Could you check a few things on this model? Use its own coordinates, in mm. A direction names the side the tool comes from. Round coordinates to 2 decimals unless told otherwise and drop trailing zeros. Loops run counter-clockwise (first coordinate to the right, second up) from the corner with the lowest first, then second, coordinate; pieces in that order, holes last. Notation, with made-up numbers: (40, -10) -> (83, -10) arc R5 ccw to (83, -6) -> close; hole circle Ø1 at (25, 40.25). An arc over 180 degrees is marked (long way). Write each question's results on one line, items separated by ' | '.
from build123d import *

# Parameters (mm, degrees)
F0_R      = 29.21
F10_DEPTH = 19.05
F1_R      = 3.175
F2_DEPTH  = 3.175
F3_R      = 1.5875
F4_DEPTH  = 28.575
F5_R      = 3.175
F11_DEPTH = 9.526
F6_R      = 1.5875
F7_DEPTH  = 25.4
F8_R      = 1.5875
F9_DEPTH  = 25.4


with BuildPart() as f10:
    # F0 (on Top) → F10 (new body)
    with BuildSketch(Plane.XY):
        with BuildLine():
            Line((38.1, 63.5), (-139.7, 63.5))
            ThreePointArc((-139.7, 63.5), (-157.6605122421, 56.0605122421), (-165.1, 38.1))
            Line((-165.1, 38.1), (-165.1, -38.1))
            ThreePointArc((-165.1, -38.1), (-157.6605122421, -56.0605122421), (-139.7, -63.5))
            Line((-139.7, -63.5), (38.1, -63.5))
            ThreePointArc((38.1, -63.5), (56.0605122421, -56.0605122421), (63.5, -38.1))
            Line((63.5, -38.1), (63.5, 6.1400658214))
            ThreePointArc((63.5, 6.1400658214), (63.1105704313, 8.3296091832), (61.9900472022, 10.2505941427))
            Line((61.9900472022, 10.2505941427), (50.937113555, 23.2651548983))
            ThreePointArc((50.937113555, 23.2651548983), (50.192630832, 25.5783429328), (51.3018729955, 27.7404426601))
            Line((51.3018729955, 27.7404426601), (61.058563678, 36.026550563))
            ThreePointArc((61.058563678, 36.026550563), (62.8898833704, 38.6267446044), (63.2307138089, 41.7887970203))
            ThreePointArc((63.2307138089, 41.7887970203), (62.4610549959, 45.2902016304), (61.206100491, 48.648370495))
            Line((61.206100491, 48.648370495), (35.46918169, 26.7906634902))
            ThreePointArc((35.46918169, 26.7906634902), (-34.6889292719, -27.7935367661), (33.8803304154, 28.7736982493))
            Line((33.8803304154, 28.7736982493), (60.0039803909, 50.9598461512))
            ThreePointArc((60.0039803909, 50.9598461512), (50.719823845, 60.1431405685), (38.1, 63.5))
        make_face()
        with Locations((-107.95, 0)):
            Circle(F0_R, mode=Mode.SUBTRACT)
    extrude(amount=F10_DEPTH)

    # F1 (on face) → F2 (cut)
    with BuildSketch(Plane.XY):
        with Locations((-152.4, -50.8)):
            Circle(F1_R)
        with Locations((50.8, -50.8)):
            Circle(F1_R)
        with Locations((50.8, 50.8)):
            Circle(F1_R)
        with Locations((-152.4, 50.8)):
            Circle(F1_R)
    extrude(amount=F2_DEPTH, mode=Mode.SUBTRACT)

    # F3 (on face) → F4 (cut)
    with BuildSketch(Plane(origin=(7.8100038105, -9.1960896842, 0), x_dir=(0.7622121578, 0.6473272947, 0), z_dir=(0.6473272947, -0.7622121578, 0))):
        with Locations((63.4603030527, 9.525)):
            Circle(F3_R)
    extrude(amount=-F4_DEPTH, mode=Mode.SUBTRACT)

    # F5 (on face) → F11 (cut, through all)
    with BuildSketch(Plane(origin=(7.8100038105, -9.1960896842, 0), x_dir=(0.7622121578, 0.6473272947, 0), z_dir=(0.6473272947, -0.7622121578, 0))):
        with Locations((63.4603030527, 9.525)):
            Circle(F5_R)
    extrude(amount=-F11_DEPTH, mode=Mode.SUBTRACT)

    # F6 (on face) → F7 (cut)
    with BuildSketch(Plane.XZ.offset(63.5)):
        with Locations((-108.2258597016, 9.525)):
            Circle(F6_R)
    extrude(amount=-F7_DEPTH, mode=Mode.SUBTRACT)

    # F8 (on face) → F9 (cut)
    with BuildSketch(Plane(origin=(-165.1, 0, 0), x_dir=(0, -1, 0), z_dir=(-1, 0, 0))):
        with Locations((0, 9.525)):
            Circle(F8_R)
    extrude(amount=-F9_DEPTH, mode=Mode.SUBTRACT)


solid = f10.part
1) I need wall thicknesses on line 1 (Y direction, x = -152.4, z = 2.3) (3 decimals); line 2 (X direction, y = 18.5, z = 1.25); line 3 (Z direction, x = -154.5, y = 0). Which ranges of each line are inside material? Lowest first, please.
Model answer:
line 1: y = -60.097 to -53.975, -47.625 to 47.625, 53.975 to 60.097 | line 2: x = -165.1 to -130.55, -85.35 to -40.42, 40.42 to 54.98 | line 3: z = 0 to 7.94, 11.11 to 19.05
2) I'm going to push flat-ended pins straight in: pin 1 (10 mm diameter, centred on x = -152.4, y = -50.8, fed in from -Z); pin 2 (6 mm diameter, centred on x = -29.5, y = -26.5, fed in from -Z); pin 3 (1.6 mm diameter, centred on y = -0.5, z = 9.5, fed in from -X); pin 4 (3 mm diameter, centred on x = -151.5, y = -51.5, fed in from -Z) (3 decimals). Where does each tip first touch, or does it pass through?
Model answer:
pin 1: stops at z = 0 | pin 2: passes through | pin 3: stops at x = -139.7 | pin 4: stops at z = 3.175
3) I want a section at D-D, the plane y = -34.5. Write out the boundary of the cut face in (x, z).
Model answer:
outline: (-165.1, 0) -> (-28.03, 0) -> (-28.03, 19.05) -> (-165.1, 19.05) -> close; (28.03, 0) -> (63.5, 0) -> (63.5, 19.05) -> (28.03, 19.05) -> close
4) If we mould it in two halves opening along X, with no side actions, what happens to faces 1 (the flat face through (-52, 1, 0)), 2 (the flat face through (51, -51, 3.175)), 3 (the flat face through (63.5, -16, 9)), 4 (the flat face through (46.76, 39.71, 9.39))? For each: released by +X, released by -X, zero draft, split by the parting line, or undercut.
Model answer:
face 1: zero draft | face 2: undercut | face 3: released by +X | face 4: undercut
5) I want a section at A-A, the plane z = 15.5. Write out the boundary of the cut face in (x, y) (3 decimals), plus the area to 3 significant figures.
Model answer:
outline: (-165.1, -38.1) arc R25.4 ccw to (-139.7, -63.5) -> (38.1, -63.5) arc R25.4 ccw to (63.5, -38.1) -> (63.5, 6.14) arc R6.35 ccw to (61.99, 10.251) -> (50.937, 23.265) arc R3.175 cw to (51.302, 27.74) -> (61.059, 36.027) arc R6.35 ccw to (63.231, 41.789) arc R25.4 ccw to (61.206, 48.648) -> (35.469, 26.791) arc R44.45 cw (long way) to (33.88, 28.774) -> (60.004, 50.96) arc R25.4 ccw to (38.1, 63.5) -> (-139.7, 63.5) arc R25.4 ccw to (-165.1, 38.1) -> close; hole circle Ø58.42 at (-107.95, 0) | area: 19,300 mm2
6) For faces 5 (the cylindrical face through (-157.46, 56.26, 9.39)), 6 (the flat face through (56.54, 16.67, 9.39)), 7 (the cylindrical face through (52.507, -48.123, 1.565)), which set-ups out of +Z, -Z, +X, -X, +Y, -Y let a thin tool reach every point of the face, with its end or its side?
Model answer:
face 5: +Z, -Z, -X, +Y | face 6: +Z, -Z, +X | face 7: -Z
7) I want a section at B-B, the plane y = 13.5. Write out the boundary of the cut face in (x, z), plus the area to 3 significant figures.
Model answer:
outline: (-165.1, 0) -> (-133.85, 0) -> (-133.85, 19.05) -> (-165.1, 19.05) -> close; (-82.05, 0) -> (-42.35, 0) -> (-42.35, 19.05) -> (-82.05, 19.05) -> close; (42.35, 0) -> (59.23, 0) -> (59.23, 19.05) -> (42.35, 19.05) -> close | area: 1,670 mm2
8) I want a section at C-C, the plane x = -35. Write out the boundary of the cut face in (y, z).
Model answer:
outline: (-63.5, 0) -> (-27.4, 0) -> (-27.4, 19.05) -> (-63.5, 19.05) -> close; (27.4, 0) -> (63.5, 0) -> (63.5, 19.05) -> (27.4, 19.05) -> close
